from build123d import *

# Parameters (mm, degrees)
BOSS_EXTRUDE1_DEPTH = 80
SKETCH3_W           = 299
SKETCH3_H           = 299
BOSS_EXTRUDE2_DEPTH = 2
SKETCH4_W           = 82
SKETCH4_H           = 299
BOSS_EXTRUDE3_DEPTH = 2
SKETCH6_W           = 299
SKETCH6_H           = 150.5
CUT_EXTRUDE1_DEPTH  = 82
SKETCH7_W           = 132
SKETCH7_H           = 2
BOSS_EXTRUDE4_DEPTH = 80
SKETCH8_R           = 1.6
CUT_EXTRUDE2_DEPTH  = 2
SKETCH12_W          = 13
SKETCH12_H          = 5
CUT_EXTRUDE4_DEPTH  = 2
SKETCH14_W          = 18
SKETCH14_H          = 11
SKETCH14_W_2        = 14
SKETCH14_H_2        = 7
BOSS_EXTRUDE5_DEPTH = 10
BOSS_EXTRUDE6_DEPTH = 30
SKETCH16_W          = 80
SKETCH16_H          = 2
BOSS_EXTRUDE7_DEPTH = 30


with BuildPart() as part:
    # Sketch1 → Boss-Extrude1 (new body)
    with BuildSketch(Plane(origin=(0, 0, 0), x_dir=(0, 0, -1), z_dir=(1, 0, 0))):
        Polygon((-23.931657395, -26.597399746), (-23.931657395, 6.402600254), (9.068342605, 6.402600254), (9.068342605, 39.402600254), (42.068342605, 39.402600254), (42.068342605, 72.402600254), (75.068342605, 72.402600254), (75.068342605, 105.402600254), (108.068342605, 105.402600254), (108.068342605, 138.402600254), (141.068342605, 138.402600254), (141.068342605, 171.402600254), (174.068342605, 171.402600254), (174.068342605, 204.402600254), (207.068342605, 204.402600254), (207.068342605, 237.402600254), (240.068342605, 237.402600254), (240.068342605, 272.402600254), (238.068342605, 272.402600254), (238.068342605, 239.402600254), (205.068342605, 239.402600254), (205.068342605, 206.402600254), (172.068342605, 206.402600254), (172.068342605, 173.402600254), (139.068342605, 173.402600254), (139.068342605, 140.402600254), (106.068342605, 140.402600254), (106.068342605, 107.402600254), (73.068342605, 107.402600254), (73.068342605, 74.402600254), (40.068342605, 74.402600254), (40.068342605, 41.402600254), (7.068342605, 41.402600254), (7.068342605, 8.402600254), (-25.931657395, 8.402600254), (-25.931657395, -24.597399746), (-58.931657395, -24.597399746), (-58.931657395, -26.597399746), align=None)
    extrude(amount=BOSS_EXTRUDE1_DEPTH)

    # Sketch3 → Boss-Extrude2 (add)
    with BuildSketch(Plane.ZY):
        with Locations((-90.568342605, 122.902600254)):
            Rectangle(SKETCH3_W, SKETCH3_H)
    extrude(amount=BOSS_EXTRUDE2_DEPTH)

    # Sketch4 → Boss-Extrude3 (add)
    with BuildSketch(Plane.XZ.offset(26.597399746)):
        with Locations((39, -90.568342605)):
            Rectangle(SKETCH4_W, SKETCH4_H)
    extrude(amount=BOSS_EXTRUDE3_DEPTH)

    # Sketch6 → Cut-Extrude1 (cut)
    with BuildSketch(Plane.ZY.offset(2)):
        with Locations((-90.568342605, 46.652600254)):
            Rectangle(SKETCH6_W, SKETCH6_H)
    extrude(amount=-CUT_EXTRUDE1_DEPTH, mode=Mode.SUBTRACT)

    # Sketch7 → Boss-Extrude4 (add)
    with BuildSketch(Plane(origin=(0, 0, 0), x_dir=(0, 0, -1), z_dir=(1, 0, 0))):
        with Locations((174.068342605, 122.902600254)):
            Rectangle(SKETCH7_W, SKETCH7_H)
    extrude(amount=BOSS_EXTRUDE4_DEPTH)

    # Sketch8 → Cut-Extrude2 (cut)
    with BuildSketch(Plane(origin=(0, 0, 0), x_dir=(0, 0, -1), z_dir=(1, 0, 0))):
        with Locations((101.068342605, 126.902600254)):
            Circle(SKETCH8_R)
        with Locations((134.068342605, 145.402600254)):
            Circle(SKETCH8_R)
        with Locations((167.068342605, 178.402600254)):
            Circle(SKETCH8_R)
        with Locations((200.068342605, 211.402600254)):
            Circle(SKETCH8_R)
        with Locations((233.068342605, 244.402600254)):
            Circle(SKETCH8_R)
    extrude(amount=-CUT_EXTRUDE2_DEPTH, mode=Mode.SUBTRACT)

    # Sketch12 → Cut-Extrude4 (cut)
    with BuildSketch(Plane.XY.offset(-238.068342605)):
        with Locations((40, 249.902600254)):
            Rectangle(SKETCH12_W, SKETCH12_H)
    extrude(amount=-CUT_EXTRUDE4_DEPTH, mode=Mode.SUBTRACT)

    # Sketch14 → Boss-Extrude5 (add)
    with BuildSketch(Plane.XY.offset(-238.068342605)):
        with Locations((40, 249.902600254)):
            Rectangle(SKETCH14_W, SKETCH14_H)
        with Locations((40, 249.902600254)):
            Rectangle(SKETCH14_W_2, SKETCH14_H_2, mode=Mode.SUBTRACT)
    extrude(amount=-BOSS_EXTRUDE5_DEPTH)

    # Sketch15 → Boss-Extrude6 (add)
    with BuildSketch(Plane(origin=(0, 0, -240.068342605), x_dir=(-1, 0, 0), z_dir=(0, 0, -1))):
        Polygon((-80, 272.402600254), (2, 272.402600254), (2, 121.902600254), (0, 121.902600254), (0, 270.402600254), (-80, 270.402600254), align=None)
    extrude(amount=BOSS_EXTRUDE6_DEPTH)

    # Sketch16 → Boss-Extrude7 (add)
    with BuildSketch(Plane(origin=(0, 0, -240.068342605), x_dir=(-1, 0, 0), z_dir=(0, 0, -1))):
        with Locations((-40, 122.902600254)):
            Rectangle(SKETCH16_W, SKETCH16_H)
    extrude(amount=BOSS_EXTRUDE7_DEPTH)


solid = part.part
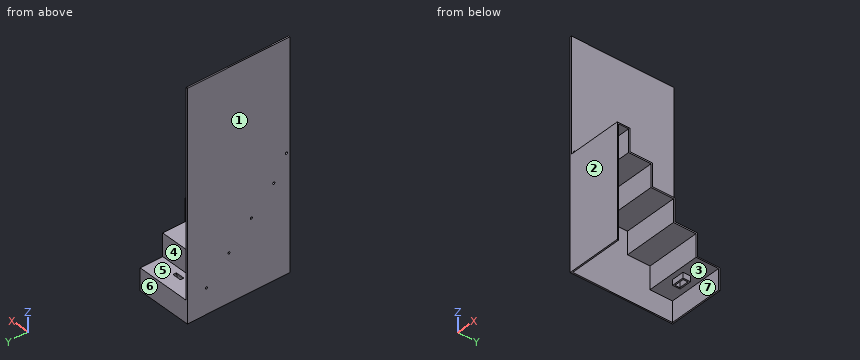
Source: CAD feature listing. Evaluate the final solid. Frame: model axes, mm. Face numbers are marked on the shaded views. A direction names the side the tool comes from. Coordinates: 2 decimals unless noted, no trailing zeros. Loops run counter-clockwise (first coordinate to the right, second up) from the corner with the lowest first, then second, coordinate; pieces in that order, holes last. Notation, with made-up numbers: M 21,24.5 L 71,24.5 A13 cw 71,46.5 Z; hole C -16,88 d7. An arc over 180 degrees is marked long. Answer in a Markdown table with one row per item.
Q1. Ray query, probe 1 along Y at (x, z) = (64.5, -225); probe 2 along Y at (x, z) = (51.5, -138); probe 3 along Z at (x, y) = (48.5, 192). Return the intervals inside material, ascending. Write a range as from..to.
Answers below:
| item | result |
|---|---|
| probe 1 | y = 121.9..123.9, 237.4..239.4 |
| probe 2 | y = 121.9..123.9, 138.4..140.4 |
| probe 3 | z = -174.07..-172.07 |
Q2. Section D-D on z = -64.5. Return the cut outline in (x, y), plus the area to 3 significant figures.
Answers below:
| item | result |
|---|---|
| outline | M -2,121.9 L 0,121.9 L 0,272.4 L -2,272.4 Z |
| area | 301 mm^2 |
Q3. First-contact query: pin 1 (4.5 mm diameter, centred on x = 38.5, y = 131.5, fed in from -Z); pin 2 (6 mm diameter, centred on x = 14.5, y = 205.5, fed in from +Z); pin 3 (16.5 mm diameter, centred on x = 48.5, z = -128, fed in from +Y); pin 4 (5 mm diameter, centred on y = 219, z = -208.5, fed in from +X). Flat tips, straight axial feed; report the tip coordinate or a pass-through.
Answers below:
| item | result |
|---|---|
| pin 1 | stops at z = -108.07 |
| pin 2 | stops at z = -172.07 |
| pin 3 | stops at y = 140.4 |
| pin 4 | stops at x = 80 |
Q4. Section B-B on z = -128. Return the cut outline in (x, y).
Answers below:
| item | result |
|---|---|
| outline | M -2,121.9 L 80,121.9 L 80,123.9 L 0,123.9 L 0,138.4 L 80,138.4 L 80,140.4 L 0,140.4 L 0,272.4 L -2,272.4 Z |
Q5. Draft query along Y for the marked faces 1, 2, 3 and 4. Return one class per face: pulls with the +Y half, pulls with the -Y half, needs draft (parallel to the pull), parting line crosses it, or undercut.
Answers below:
| item | result |
|---|---|
| face 1 | needs draft |
| face 2 | pulls with the -Y half |
| face 3 | undercut |
| face 4 | pulls with the +Y half |
Q6. Set-up query: the marked faces 5, 6 and 7. Return all of +Z, -Z, +X, -X, +Y, -Y with unobstructed straight access to the full face (end or side cutting, diameter ignored); none if empty.
Answers below:
| item | result |
|---|---|
| face 5 | +Z, +X, +Y |
| face 6 | +Z, -Z, +X, -X, +Y |
| face 7 | -Z, +X |
Q7. Section C-C on x = 67. Return the cut outline in (y, z), plus the area to 3 significant figures.
Answers below:
| item | result |
|---|---|
| outline | M 121.9,-270.07 L 123.9,-270.07 L 123.9,-108.07 L 138.4,-108.07 L 138.4,-141.07 L 171.4,-141.07 L 171.4,-174.07 L 204.4,-174.07 L 204.4,-207.07 L 237.4,-207.07 L 237.4,-240.07 L 270.4,-240.07 L 270.4,-270.07 L 272.4,-270.07 L 272.4,-238.07 L 239.4,-238.07 L 239.4,-205.07 L 206.4,-205.07 L 206.4,-172.07 L 173.4,-172.07 L 173.4,-139.07 L 140.4,-139.07 L 140.4,-106.07 L 121.9,-106.07 Z |
| area | 949 mm^2 |
Q8. Section A-A on y = 232. Return the cut outline in (x, z).
Answers below:
| item | result |
|---|---|
| outline | M -2,-270.07 L 0,-270.07 L 0,-207.07 L 80,-207.07 L 80,-205.07 L 0,-205.07 L 0,58.93 L -2,58.93 Z |
